from build123d import *

# Parameters (mm, degrees)
SKETCH_1_W          = 250
SKETCH_1_H          = 29
EXTRUDE_1_DEPTH     = 10
SKETCH_1_3_R        = 3.1
CUT_EXTRUDE_1_DEPTH = 127.234900087
SKETCH_3_W          = 20
SKETCH_3_H          = 29
EXTRUDE_2_DEPTH     = 3
SKETCH_4_W          = 53
SKETCH_4_H          = 17
SKETCH_4_R          = 3.1
EXTRUDE_3_DEPTH     = 5


with BuildPart() as part:
    # 草图1 → 凸台-拉伸1 (new body)
    with BuildSketch(Plane(origin=(0, 0, 0), x_dir=(0, 0, -1), z_dir=(1, 0, 0))):
        Rectangle(SKETCH_1_W, SKETCH_1_H)
    extrude(amount=EXTRUDE_1_DEPTH)

    # 草图1<3> → 切除-拉伸1 (cut, through all)
    with BuildSketch(Plane(origin=(0, 0, 0), x_dir=(0, 0, -1), z_dir=(1, 0, 0))):
        with Locations((-90, -10.858617882)):
            Circle(SKETCH_1_3_R)
        with Locations((-30, -10.858617882)):
            Circle(SKETCH_1_3_R)
        with Locations((30, -10.858617882)):
            Circle(SKETCH_1_3_R)
        with Locations((-60, 10.858617882)):
            Circle(SKETCH_1_3_R)
        with Locations((90, -10.858617882)):
            Circle(SKETCH_1_3_R)
        with Locations((0, 10.858617882)):
            Circle(SKETCH_1_3_R)
        with Locations((60, 10.858617882)):
            Circle(SKETCH_1_3_R)
    extrude(amount=CUT_EXTRUDE_1_DEPTH, mode=Mode.SUBTRACT)

    # 草图3 → 凸台-拉伸2 (add)
    with BuildSketch(Plane(origin=(10, 0, 0), x_dir=(0, 0, -1), z_dir=(1, 0, 0))):
        with Locations((115, 0)):
            Rectangle(SKETCH_3_W, SKETCH_3_H)
        with Locations((-115, 0)):
            Rectangle(SKETCH_3_W, SKETCH_3_H)
    extrude(amount=EXTRUDE_2_DEPTH)

    # 草图4 → 凸台-拉伸3 (add)
    # profile 1 of 2: a face of its own
    with BuildSketch(Plane(origin=(13, 0, 0), x_dir=(0, 0, -1), z_dir=(1, 0, 0))):
        with Locations((131.5, 0)):
            Rectangle(SKETCH_4_W, SKETCH_4_H)
        with Locations((150, 0)):
            Circle(SKETCH_4_R, mode=Mode.SUBTRACT)
    # profile 2 of 2: a face of its own
    with BuildSketch(Plane(origin=(13, 0, 0), x_dir=(0, 0, -1), z_dir=(1, 0, 0))):
        with Locations((-131.5, 0)):
            Rectangle(SKETCH_4_W, SKETCH_4_H)
        with Locations((-150, 0)):
            Circle(SKETCH_4_R, mode=Mode.SUBTRACT)
    extrude(amount=EXTRUDE_3_DEPTH)


solid = part.part
Can you work these out from the model? Positions are in its coordinate system, mm. A direction names the side the tool comes from. Coordinates: 2 decimals unless noted, no trailing zeros. Order: outer loops, then holes, each group sorted by start corner. A loop starts at its lowest first (then second) coordinate and runs counter-clockwise, first axis right, second up. Notation, with made-up numbers: (19, -20.75) - (67, -20.75) arc R16 ccw to (67, -9.75) - close; hole circle Ø10 at (62.5, 8.25). An arc over 180 degrees is marked (long way). Answer as a JSON object with one key per item and string values. Group by question number.
Q1. Will these pins go through, and if not, where does the flat tip stop? P1, Ø2.5, axis at x = 15, z = -119, coming from the +Y side; P2, Ø6.5, axis at x = 5.5, y = -6.5, coming from the -Z side; P3, Ø5, axis at y = -10.86, z = 30, coming from the -X side; P4, Ø2.5, axis at x = 15, z = -132.5, coming from the -Y side.
Q2. We'd pull the mould along Z, two halves only. Please class faces 6 (the face through (15, 0, 158)), 7 (the face through (15.465, 0.931, 147.043)), 8 (the face through (5, -14.5, 2)): +Z half, -Z half, draft (parallel to the pull), parting line (faces both ways), or undercut.
Q3. Imagine slicing it at B-B (z = 119.5). Please give me the cut outline in (x, y).
Q4. Imagine slicing it at A-A (z = -150). Please give me the cut outline in (x, y), and give its area (3 significant figures).
Q5. On a 3-axis mill with a long thin cutter (end or side, diameter ignored), from which of +Z, -Z, +X, -X, +Y, -Y can I reach the whole of each face in a straight line? I mean faces 1 (the face through (10, 0, 1)), 2 (the face through (13, 12, 115)), 3 (the face through (4.93, -9.927, -92.957)), 4 (the face through (15, -8.5, -131)), 5 (the face through (5, 14.5, 2)). Say none if no direction works.
Q6. Imagine slicing it at C-C (z = 0). Please give me the cut outline in (x, y), and give its area (3 significant figures).
Q7. I need wall thicknesses on line 1 (Y direction, x = 7, z = 60); line 2 (Z direction, x = 11, y = 3.5); line 3 (Z direction, x = 16.25, y = 4). Which ranges of each line are inside material? Lowest first, please. Write a range as from..to.
Determined:
{
 "1": {"P1": "stops at y = 8.5", "P2": "stops at z = -125", "P3": "passes through", "P4": "stops at y = -8.5"},
 "2": {"face 6": "+Z half", "face 7": "undercut", "face 8": "draft"},
 "3": {"outline": "(0, -14.5) - (13, -14.5) - (13, -8.5) - (18, -8.5) - (18, 8.5) - (13, 8.5) - (13, 14.5) - (0, 14.5) - close"},
 "4": {"outline": "(13, -8.5) - (18, -8.5) - (18, -3.1) - (13, -3.1) - close; (13, 3.1) - (18, 3.1) - (18, 8.5) - (13, 8.5) - close", "area": "54.0 mm2"},
 "5": {"face 1": "+X, +Y, -Y", "face 2": "+Z, -Z, +X, +Y", "face 3": "+X, -X", "face 4": "+Z, -Z, +X, -Y", "face 5": "+Z, -Z, +X, -X, +Y"},
 "6": {"outline": "(0, -14.5) - (10, -14.5) - (10, 7.76) - (0, 7.76) - close; (0, 13.96) - (10, 13.96) - (10, 14.5) - (0, 14.5) - close", "area": "228 mm2"},
 "7": {"line 1": "y = -14.5..7.76, 13.96..14.5", "line 2": "z = -125..-105, 105..125", "line 3": "z = -158..-105, 105..158"}
}
